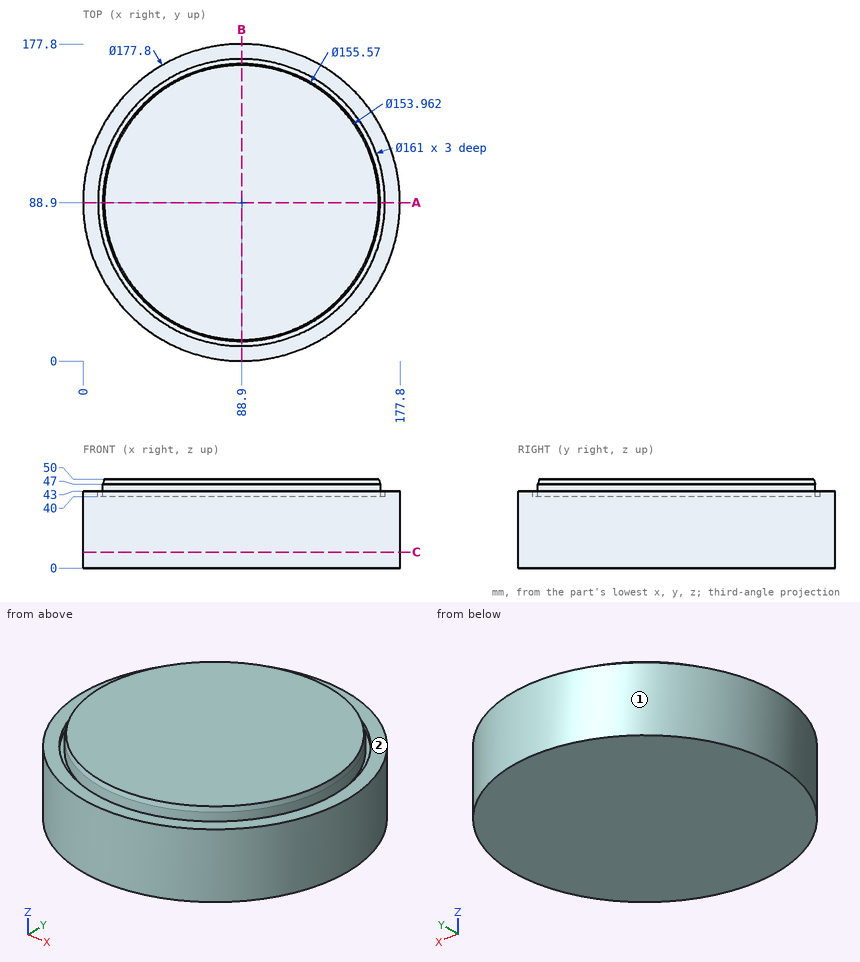
Geometry: see drawing. Coordinates: mm, zero at the bounding-box minimum. A direction names the side the tool comes from. Give positions to 0.01 mm unless a question says otherwise; leave off trailing zeros. Write each loop counter-clockwise with the first axis right and the second up, starting at its lowest first coordinate (ties: lowest second). Pieces come first, ordered by that corner, then holes. Notation, with made-up numbers: M 70.5,69 L 95.5,69 A20 ccw 95.5,100 Z; hole C 8,-14 d1. An arc over 180 degrees is marked long. Answer as a JSON object with one key per item and string values.
Q1. Contact query for flat-ended pins moving along their axis: P1, Ø1.5, axis at y = 120, z = 19, coming from the +X side; P2, Ø5, axis at y = 131, z = 41.5, coming from the +X side; P3, Ø10, axis at x = 117, z = 21.5, coming from the -Y side. Output: stop coordinate, or through.
Geometry check:
{"P1": "stops at x = 172.46", "P2": "stops at x = 168.49", "P3": "stops at y = 3.05"}
Q2. Cut plane A-A, the plane y = 88.9. Return the cut outline in (x, z) (1 decimal).
Geometry check:
{"outline": "M 0,0 L 177.8,0 L 177.8,43 L 169.4,43 L 169.4,40 L 166.7,40 L 166.7,47 L 165.9,50 L 11.9,50 L 11.1,47 L 11.1,40 L 8.4,40 L 8.4,43 L 0,43 Z"}
Q3. Access query for the marked faces 1 and 2. Directions: +Z, -Z, +X, -X, +Y, -Y. A direction counts if a zero-diameter tool reaches every point of the face in a straight line with its end or side. Return the directions, or none.
Geometry check:
{"face 1": "+Z, -Z", "face 2": "+Z"}
Q4. Cut plane C-C, the plane z = 9. Return the cut outline in (x, y).
Geometry check:
{"outline": "C 88.9,88.9 d177.8"}
Q5. Ray query, line 1 along Y through (x, z) = (88.9, 41.7) (1 decimal); line 2 along X through (y, z) = (132, 42.5). Return the intervals inside material, ascending.
Geometry check:
{"line 1": "y = 0 to 8.4, 11.1 to 166.7, 169.4 to 177.8", "line 2": "x = 11.15 to 20.91, 24.15 to 153.65, 156.89 to 166.65"}
